Model file for the job. Use its own axes, mm. Face numbers are marked on the shaded views. A direction names the side the tool comes from. Give positions to 0.01 mm unless a question says otherwise; leave off trailing zeros. Order: outer loops, then holes, each group sorted by start corner. A loop starts at its lowest first (then second) coordinate and runs counter-clockwise, first axis right, second up. Notation, with made-up numbers: M 28.5,44 L 87.5,44 A21 ccw 87.5,81 Z; hole C 34.25,-35.5 d11. An arc over 180 degrees is marked long. Return JSON: item names as keys, results as strings. Group by question number.
1. 3-axis set-ups, long thin cutter, end or side, ignore diameter. For the marked faces 1 and 2: which of +Z, -Z, +X, -X, +Y, -Y reach the whole face in a straight line?
2. Slice it at A-A on y = 0. List the corners of the cut face in (x, z).
3. Slice it at D-D on z = 17. List the corners of the cut face in (x, y).
4. Slice it at C-C on z = 5.25. List the corners of the cut face in (x, y).
5. Pin check, flat tips, straight feed: pin 1 (8 mm diameter, centred on x = -19.5, z = 16.5, fed in from -Y); pin 2 (1.5 mm diameter, centred on x = -9, y = -19, fed in from -Z); pin 3 (1.5 mm diameter, centred on y = -9, z = 6.5, fed in from -X). Stop position of each tip, or through.
6. Wall check: probe 1 along Y at (x, z) = (0, 14.5); probe 2 along X at (y, z) = (0, 4.8); probe 3 along Z at (x, y) = (-7.5, 6). Give the ranges that are in metal, low to high. Write a range as [from, to].
7. Two-plate mould, pull along X, no slides. Class the marked faces 3, 4, 5 and 6: released by +X, released by -X, zero draft, split by the parting line, or undercut.
from build123d import *

# Parameters (mm, degrees)
SKETCH_R        = 37.5
PAD_DEPTH       = 20
SKETCH001_R     = 41.795257
SKETCH001_R_2   = 31
POCKET_DEPTH    = 8
SKETCH002_R     = 43.633229
SKETCH002_R_2   = 35
POCKET001_DEPTH = 8
SKETCH003_R     = 30
POCKET002_DEPTH = 8
SKETCH004_R     = 4
POCKET003_DEPTH = 20
FILLET_R        = 2


with BuildPart() as part:
    # Sketch → Pad (new body)
    with BuildSketch(Plane.XY):
        Circle(SKETCH_R)
    extrude(amount=PAD_DEPTH)

    # Sketch001 (on Face3 of Pad) → Pocket (cut)
    with BuildSketch(Plane.XY.offset(20)):
        Circle(SKETCH001_R)
        Circle(SKETCH001_R_2, mode=Mode.SUBTRACT)
    extrude(amount=-POCKET_DEPTH, mode=Mode.SUBTRACT)

    # Sketch002 (on Face2 of Pocket) → Pocket001 (cut)
    with BuildSketch(Plane(origin=(0, 0, 0), x_dir=(1, 0, 0), z_dir=(0, 0, -1))):
        Circle(SKETCH002_R)
        Circle(SKETCH002_R_2, mode=Mode.SUBTRACT)
    extrude(amount=-POCKET001_DEPTH, mode=Mode.SUBTRACT)

    # Sketch003 (on Face6 of Pocket001) → Pocket002 (cut)
    with BuildSketch(Plane(origin=(0, 0, 0), x_dir=(1, 0, 0), z_dir=(0, 0, -1))):
        Circle(SKETCH003_R)
    extrude(amount=-POCKET002_DEPTH, mode=Mode.SUBTRACT)

    # Sketch004 (on Face7 of Pocket002) → Pocket003 (cut)
    with BuildSketch(Plane.XY.offset(20)):
        Circle(SKETCH004_R)
    extrude(amount=-POCKET003_DEPTH, mode=Mode.SUBTRACT)

    # Fillet
    fillet_edges = [part.edges().sort_by_distance(p)[0] for p in [
        (-31, 0, 20),
        (-37.5, 0, 12),
        (-30, 0, 0),
        (-35, 0, 0),
    ]]
    fillet(fillet_edges, radius=FILLET_R)


solid = part.part
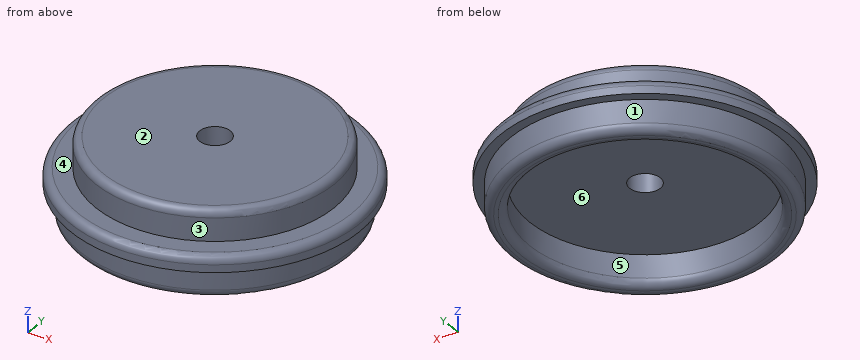
Result:
{
 "1": {"face 1": "-Z", "face 2": "+Z, +X, -X, +Y, -Y"},
 "2": {"outline": "M -37.5,8 L -35,8 L -35,2 A2 ccw -33,0 L -32,0 A2 ccw -30,2 L -30,8 L -4,8 L -4,20 L -29,20 A2 ccw -31,18 L -31,12 L -35.5,12 A2 ccw -37.5,10 Z; M 4,8 L 30,8 L 30,2 A2 ccw 32,0 L 33,0 A2 ccw 35,2 L 35,8 L 37.5,8 L 37.5,10 A2 ccw 35.5,12 L 31,12 L 31,18 A2 ccw 29,20 L 4,20 Z"},
 "3": {"outline": "C 0,0 d62; hole C 0,0 d8"},
 "4": {"outline": "C 0,0 d70; hole C 0,0 d60"},
 "5": {"pin 1": "stops at y = -26.85", "pin 2": "stops at z = 8", "pin 3": "stops at x = -34.01"},
 "6": {"probe 1": "y = [-31, -4], [4, 31]", "probe 2": "x = [-35, -30], [30, 35]", "probe 3": "z = [8, 20]"},
 "7": {"face 3": "split by the parting line", "face 4": "zero draft", "face 5": "undercut", "face 6": "undercut"}
}
